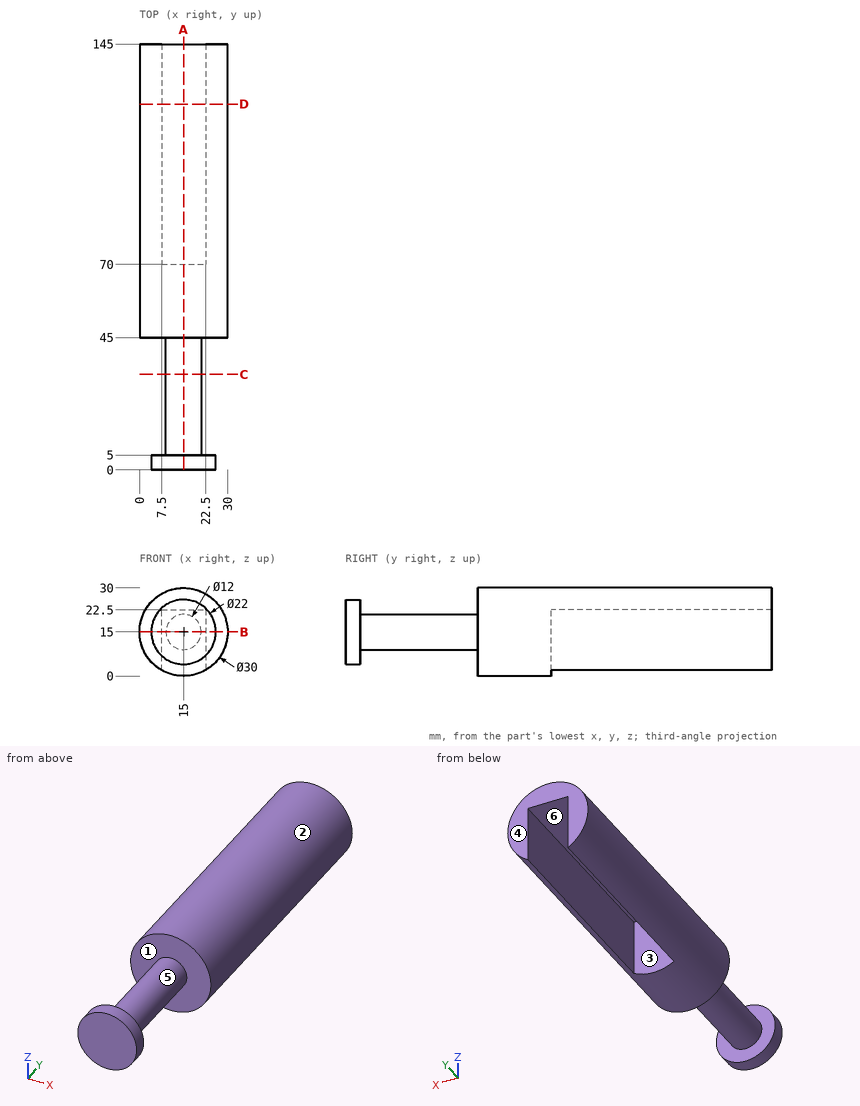
Verification items for this drawing (mm, ordinates from the low corner). A direction names the side the tool comes from. Give positions to 0.01 mm unless a question says otherwise; leave off trailing zeros. Loops run counter-clockwise (first coordinate to the right, second up) from the corner with the lowest first, then second, coordinate; pieces in that order, holes last. Notation, with made-up numbers: M 44.5,-34 L 78.5,-34 A14 ccw 78.5,-22 Z; hole C 83.25,75 d3. An arc over 180 degrees is marked long. Answer as a JSON object with one key per item and string values. Group by question number.
Q1. Release check for a two-part mould opening along Y. For the marked faces 4, 5 and 6 record: released by +Y, released by -Y, zero draft, split by the parting line, or undercut.
Q2. Material ranges on line 1 along Y through (x, z) = (14.5, 7); line 2 along Y through (x, z) = (13.75, 25); line 3 along Y through (x, z) = (8.75, 24.25), recorded low to high. Write a range as [from, to].
Q3. Access from +Z, -Z, +X, -X, +Y, -Y to the whole of each face (thin tool, end or side, straight path). Record for the marked faces 1, 2 and 3.
Q4. Cross-section at A-A on x = 15. Record the cut outline in (y, z).
Q5. Cross-section at C-C on y = 32.5. Record the cut outline in (x, z).
Q6. Cross-section at B-B on z = 15. Record the cut outline in (x, y), then the cut area to 4 significant figures.
Q7. Cross-section at D-D on y = 124.5. Record the cut outline in (x, z), then the cut area to 3 significant figures.
Q8. Go/stop test with flat-tipped pins: P1, Ø4.5, axis at x = 16, y = 109, coming from the -Z side; P2, Ø4.5, axis at x = 16, z = 13.5, coming from the +Y side; P3, Ø12, axis at x = 22.5, y = 24.5, coming from the -Z side. Record where each tip stops, or that it passes through.
Evaluation:
{
 "1": {"face 4": "released by +Y", "face 5": "undercut", "face 6": "zero draft"},
 "2": {"line 1": "y = [0, 5], [45, 70]", "line 2": "y = [0, 5], [45, 145]", "line 3": "y = [45, 145]"},
 "3": {"face 1": "none", "face 2": "+Y, -Y", "face 3": "-Z, +Y"},
 "4": {"outline": "M 0,4 L 5,4 L 5,9 L 45,9 L 45,0 L 70,0 L 70,22.5 L 145,22.5 L 145,30 L 45,30 L 45,21 L 5,21 L 5,26 L 0,26 Z"},
 "5": {"outline": "C 15,15 d12"},
 "6": {"outline": "M 0,45 L 9,45 L 9,5 L 4,5 L 4,0 L 26,0 L 26,5 L 21,5 L 21,45 L 30,45 L 30,145 L 22.5,145 L 22.5,70 L 7.5,70 L 7.5,145 L 0,145 Z", "area": "2,465 mm2"},
 "7": {"outline": "M 7.5,2.01 L 7.5,22.5 L 22.5,22.5 L 22.5,2.01 A15 ccw long Z", "area": "379 mm2"},
 "8": {"P1": "stops at z = 22.5", "P2": "stops at y = 70", "P3": "stops at z = 9.19"}
}
